Can you work these out from the model? Positions are in its coordinate system, mm. Face numbers are marked on the shaded views. A direction names the side the tool comes from. Give positions to 0.01 mm unless a question says otherwise; leave off trailing zeros. Write each loop counter-clockwise with the first axis right and the second up, starting at its lowest first coordinate (ties: lowest second). Pieces come first, ordered by that corner, then holes. Notation, with made-up numbers: M 33.5,88.25 L 42.5,88.25 A29 cw 42.5,119.25 Z; hole C -3.5,30 d7. An arc over 180 degrees is marked long. Write each question's results on one line, items separated by ' | '.
from build123d import *

# Parameters (mm, degrees)
SKETCH1_R           = 16.625
SKETCH1_R_2         = 15.5
BOSS_EXTRUDE1_DEPTH = 15
BOSS_EXTRUDE1_DRAFT = 2
SKETCH4_R           = 18.625
SKETCH4_R_2         = 15.5
BOSS_EXTRUDE2_DEPTH = 2
SKETCH5_R           = 16.625
SKETCH5_R_2         = 15.5
BOSS_EXTRUDE3_DEPTH = 5
SKETCH9_R           = 16.101188458
SKETCH9_R_2         = 15.5
BOSS_EXTRUDE5_DEPTH = 15
BOSS_EXTRUDE8_DEPTH = 6.3
SKETCH11_R          = 3.9
CUT_EXTRUDE2_DEPTH  = 35.318817724


with BuildPart() as part:
    # Sketch1 → Boss-Extrude1 (with draft: the straight prism first)
    with BuildSketch(Plane(origin=(0, 0, 0), x_dir=(1, 0, 0), z_dir=(0, 1, 0))):
        Circle(SKETCH1_R)
        Circle(SKETCH1_R_2, mode=Mode.SUBTRACT)
    extrude(amount=BOSS_EXTRUDE1_DEPTH)
    # Boss-Extrude1: the draft: its side faces are tilted about the plane it starts from
    boss_extrude1_sides = [part.faces().sort_by_distance(p)[0] for p in [
        (-16.625, 7.5, 0),
        (-15.5, 7.5, 0),
    ]]
    draft(boss_extrude1_sides, Plane(origin=(0, 0, 0), x_dir=(1, 0, 0), z_dir=(0, 1, 0)), BOSS_EXTRUDE1_DRAFT)

    # Sketch4 → Boss-Extrude2 (add)
    with BuildSketch(Plane(origin=(0, 0, 0), x_dir=(1, 0, 0), z_dir=(0, 1, 0))):
        with Locations(Location((0, 0, 0), (0, 0, 270))):
            Circle(SKETCH4_R)
        with Locations(Location((0, 0, 0), (0, 0, 270))):
            Circle(SKETCH4_R_2, mode=Mode.SUBTRACT)
    extrude(amount=-BOSS_EXTRUDE2_DEPTH)

    # Sketch5 → Boss-Extrude3 (add)
    with BuildSketch(Plane.XZ.offset(2)):
        with Locations(Location((0, 0, 0), (0, 0, 90))):
            Circle(SKETCH5_R)
        with Locations(Location((0, 0, 0), (0, 0, 90))):
            Circle(SKETCH5_R_2, mode=Mode.SUBTRACT)
    extrude(amount=BOSS_EXTRUDE3_DEPTH)

    # Sketch9 → Boss-Extrude5 (add, through all)
    with BuildSketch(Plane(origin=(0, 0, 0), x_dir=(1, 0, 0), z_dir=(0, 1, 0))):
        Circle(SKETCH9_R)
        with Locations(Location((0, 0, 0), (0, 0, 270))):
            Circle(SKETCH9_R_2, mode=Mode.SUBTRACT)
    extrude(amount=BOSS_EXTRUDE5_DEPTH)

    # Sketch10 → Boss-Extrude8 (add)
    with BuildSketch(Plane(origin=(0, 15, 0), x_dir=(1, 0, 0), z_dir=(0, 1, 0))):
        with BuildLine():
            Line((-1.490883565, 5.294078409), (-1.490883565, 15.428132298))
            ThreePointArc((-1.490883565, 15.428132298), (0.009159426, 15.499997294), (1.509116435, 15.426359505))
            Line((1.509116435, 15.426359505), (1.509116435, 5.288909867))
            ThreePointArc((1.509116435, 5.288909867), (5.5, 0), (1.509116435, -5.288909867))
            Line((1.509116435, -5.288909867), (1.509116435, -15.426359505))
            ThreePointArc((1.509116435, -15.426359505), (0.009159426, -15.499997294), (-1.490883565, -15.428132298))
            Line((-1.490883565, -15.428132298), (-1.490883565, -5.294078409))
            ThreePointArc((-1.490883565, -5.294078409), (-5.5, 0), (-1.490883565, 5.294078409))
        make_face()
    extrude(amount=-BOSS_EXTRUDE8_DEPTH)

    # Sketch11 → Cut-Extrude2 (cut, through all)
    with BuildSketch(Plane(origin=(0, 15, 0), x_dir=(1, 0, 0), z_dir=(0, 1, 0))):
        with Locations(Location((0, 0, 0), (0, 0, 270))):
            Circle(SKETCH11_R)
    extrude(amount=-CUT_EXTRUDE2_DEPTH, mode=Mode.SUBTRACT)

    # Cut-Extrude3 cone 1 section (through the dimple's axis) → Cut-Extrude3 (revolve, cut)
    with BuildSketch(Plane(origin=(0, 15, 0), x_dir=(0, 0, 1), z_dir=(1, 0, 0))):
        Polygon((0, 0), (4.75, 0), (0, 8.227241336), align=None)
    revolve(axis=Axis((0, 15, 0), (0, -1, 0)), mode=Mode.SUBTRACT)


solid = part.part
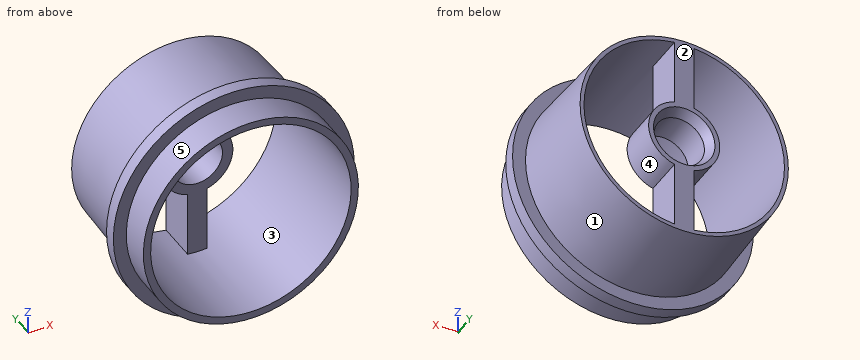
Item 1: I want a section at D-D, the plane y = 2. Please give me the cut outline in (x, z), and give its area (3 significant figures).
Geometry says:
outline: C 0,0 d33.11; hole C 0,0 d31 | area: 106 mm2
Item 2: I want a section at A-A, the plane x = 0. Please give me the cut outline in (y, z) (3 decimals).
Geometry says:
outline: M -7,-16.625 L -2,-16.625 L -2,-18.625 L 0,-18.625 L 0,-16.625 L 15,-16.101 L 15,-4.75 L 13.528,-3.9 L 8.7,-3.9 L 8.7,-15.5 L -7,-15.5 Z; M -7,15.5 L 8.7,15.5 L 8.7,3.9 L 13.528,3.9 L 15,4.75 L 15,16.101 L 0,16.625 L 0,18.625 L -2,18.625 L -2,16.625 L -7,16.625 Z
Item 3: I'm going to push flat-ended pins straight in: pin 1 (1.9 mm diameter, centred on y = 11.5, z = -8.5, fed in from -X); pin 2 (18.5 mm diameter, centred on x = 0, z = 0, fed in from +Y); pin 3 (5.5 mm diameter, centred on x = -2.5, z = 0, fed in from -Y); pin 4 (10 mm diameter, centred on y = -1, z = -5, fed in from +X) (3 decimals). Where does each tip first touch, or does it pass through?
Geometry says:
pin 1: stops at x = -14.36 | pin 2: stops at y = 15 | pin 3: stops at y = 8.7 | pin 4: stops at x = 18.625
Item 4: I want a section at B-B, the plane z = 0. Please give me the cut outline in (x, y) (3 decimals).
Geometry says:
outline: M -18.625,-2 L -16.625,-2 L -16.625,-7 L -15.5,-7 L -15.5,15 L -16.101,15 L -16.625,0 L -18.625,0 Z; M -5.5,8.7 L -3.9,8.7 L -3.9,13.528 L -4.75,15 L -5.5,15 Z; M 3.9,8.7 L 5.5,8.7 L 5.5,15 L 4.75,15 L 3.9,13.528 Z; M 15.5,-7 L 16.625,-7 L 16.625,-2 L 18.625,-2 L 18.625,0 L 16.625,0 L 16.101,15 L 15.5,15 Z
Item 5: If I drill on line 1 (X direction, y = 11.5, z = -2); line 2 (Z direction, x = -2, y = 9.5); line 3 (Y direction, x = -12.5, z = -12), over which ranges is the centre line in solid material (lowest first)? Write a range as from..to.
Geometry says:
line 1: x = -16.1..-15.37, -5.12..-3.35, 3.35..5.12, 15.37..16.1 | line 2: z = -16.17..-15.37, -5.12..-3.35, 3.35..5.12, 15.37..16.17 | line 3: y = -2..0
Item 6: Thinking about a two-plate mould opening in X: for the marked faces 1, 2 and 3, which applies, +X half, -X half, draft (parallel to the pull), parting line (faces both ways), or undercut?
Geometry says:
face 1: parting line | face 2: draft | face 3: undercut
Item 7: For the marked faces 4 and 5, which set-ups out of +Z, -Z, +X, -X, +Y, -Y let a thin tool reach every point of the face, with its end or its side?
Geometry says:
face 4: +Y, -Y | face 5: -Y
Item 8: I want a section at C-C, the plane z = -8. Give the number of separate pieces and of enclosed holes in the cut face, and give its area (3 significant figures).
Geometry says:
separate pieces: 3 | enclosed holes: 0 | area: 76.0 mm2
